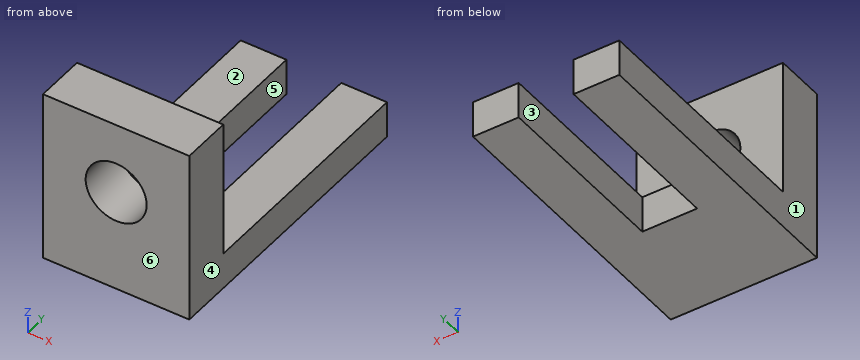
from build123d import *

# Parameters (mm, degrees)
F0_W     = 3
F0_H     = 12
F1_DEPTH = 4
F3_W     = 16
F3_H     = 5.5
F4_DEPTH = 15
F5_R     = 3.33375
F6_DEPTH = 32.001


with BuildPart() as f1:
    # F0 (on Top) → F1 (new body)
    with BuildSketch(Plane.XY):
        with Locations((1.5, 6)):
            Rectangle(F0_W, F0_H)
        Polygon((3, 12), (3, 0), (8, 0), (8, 32), (3, 32), align=None)
    extrude(amount=-F1_DEPTH)

    # F2: F1 across face


with BuildPart() as f1_1:
    add(f1.part)
    add(f1.part.mirror(Plane(origin=(0, 6, -2), x_dir=(0, -1, 0), z_dir=(-1, 0, 0))))

    # F3 (on face) → F4 (join)
    with BuildSketch(Plane.XY):
        with Locations((0, 2.75)):
            Rectangle(F3_W, F3_H)
    extrude(amount=F4_DEPTH)

    # F5 (on Front) → F6 (cut, through all)
    with BuildSketch(Plane.XZ):
        with Locations((0, 7.2)):
            Circle(F5_R)
    extrude(amount=-F6_DEPTH, mode=Mode.SUBTRACT)


solid = f1_1.part
Design review of the part built by this model. Coordinates are the model's own, in mm. Face numbers are marked on the shaded views. A direction names the side the tool comes from. Give positions to 0.01 mm unless a question says otherwise; leave off trailing zeros. Loops run counter-clockwise (first coordinate to the right, second up) from the corner with the lowest first, then second, coordinate; pieces in that order, holes last. Notation, with made-up numbers: M 69.25,5 L 110.25,5 A32 cw 110.25,37 Z; hole C 41.25,-12.5 d7. An arc over 180 degrees is marked long. One line per question, with ' | ' between items. Start each with the question number.
1. Add section D-D (z = -1.25). Write out the cut boundary in (x, y).
2. Add section B-B (z = 7.2). Write out the cut boundary in (x, y).
3. Insertion check: P1, Ø1.5, axis at x = -3.5, z = 4, coming from the -Y side; P2, Ø4.5, axis at x = 0, z = 7.5, coming from the +Y side; P3, Ø8, axis at x = -6.5, y = 27.5, coming from the +Z side; P4, Ø4, axis at x = 5.5, z = 12.5, coming from the +Y side. Each pin has a flat end and moves straight along its axis. Give the tip position at first contact, or say it passes through.
4. Add section A-A (y = 24.5). Write out the cut boundary in (x, z).
5. The part is to be moulded in two halves that separate along X. For the marked faces 4, 5 and 6, say which applies: released by +X, released by -X, zero draft, split by the parting line, or undercut.
6. Add section C-C (x = 0). Write out the cut boundary in (y, z), plus the area to 3 significant figures.
7. For the marked faces 1, 2 and 3, list the 3-axis set-ups (+Z, -Z, +X, -X, +Y, -Y) from which the entire face can be reached by the end or side of a thin tool; tool diameter is ignored.
8. To check wall thickness, follow L1, parallel to X at y = 22, z = -1; L2, parallel to Z at x = 0, y = 2.7; L3, parallel to Y at x = 5.5, z = 1.5. State the ranges of each line that lie inside material, in increasing order.
Worked out:
1) outline: M -8,0 L 8,0 L 8,32 L 3,32 L 3,12 L -3,12 L -3,32 L -8,32 Z
2) outline: M -8,0 L -3.33,0 L -3.33,5.5 L -8,5.5 Z; M 3.33,0 L 8,0 L 8,5.5 L 3.33,5.5 Z
3) P1: stops at y = 0 | P2: passes through | P3: stops at z = 0 | P4: stops at y = 5.5
4) outline: M -8,-4 L -3,-4 L -3,0 L -8,0 Z; M 3,-4 L 8,-4 L 8,0 L 3,0 Z
5) face 4: released by +X | face 5: undercut | face 6: zero draft
6) outline: M 0,-4 L 12,-4 L 12,0 L 5.5,0 L 5.5,3.87 L 0,3.87 Z; M 0,10.53 L 5.5,10.53 L 5.5,15 L 0,15 Z | area: 93.8 mm²
7) face 1: +Z, -Z, -X, +Y, -Y | face 2: +Z, +X, -X, +Y | face 3: +Z, -Z, +Y
8) L1: x = -8 to -3, 3 to 8 | L2: z = -4 to 3.87, 10.53 to 15 | L3: y = 0 to 5.5
